```python
from build123d import *

# Parameters (mm, degrees)
BOSS_EXTRUDE3_DEPTH = 4.7625
BOSS_EXTRUDE5_DEPTH = 1.5875
SKETCH12_W          = 6.35
SKETCH12_H          = 35.71875
CUT_EXTRUDE1_DEPTH  = 9.652


with BuildPart() as part:
    # Sketch1 → Boss-Extrude3 (new body)
    with BuildSketch(Plane.XY):
        Polygon((43.795067265, 15.433632287), (5.695067265, 15.433632287), (5.695067265, -60.766367713), (43.795067265, -60.766367713), (43.795067265, -25.047617713), (31.095067265, -25.047617713), (31.095067265, -20.285117713), (43.795067265, -20.285117713), align=None)
    extrude(amount=BOSS_EXTRUDE3_DEPTH)

    # Sketch3 → Boss-Extrude5 (add)
    with BuildSketch(Plane.XY.offset(4.7625)):
        Polygon((18.395067265, -6.791367713), (5.695067265, -6.791367713), (5.695067265, -22.666367713), (5.695067265, -38.541367713), (18.395067265, -38.541367713), align=None)
    extrude(amount=BOSS_EXTRUDE5_DEPTH)

    # Sketch12 → Cut-Extrude1 (cut)
    with BuildSketch(Plane.XY.offset(4.7625)):
        with Locations((40.620067265, -42.906992713)):
            Rectangle(SKETCH12_W, SKETCH12_H)
        with Locations((40.620067265, -2.425742713)):
            Rectangle(SKETCH12_W, SKETCH12_H)
    extrude(amount=-CUT_EXTRUDE1_DEPTH, mode=Mode.SUBTRACT)


solid = part.part
```
CAD build for the part. Positions are in the model's coordinates, mm. A direction names the side the tool comes from. Coordinates: 2 decimals unless noted, no trailing zeros. Loops run counter-clockwise (first coordinate to the right, second up) from the corner with the lowest first, then second, coordinate; pieces in that order, holes last. Notation, with made-up numbers: (48, 56.25) - (97, 56.25) arc R20 cw to (97, 83.25) - close; hole circle Ø1 at (53, 60.25). An arc over 180 degrees is marked (long way). Use CSV: the item, a comma, the result in double quotes. Start each with the question number.
Q1. Cut at A-A, the plane x = 35. List the corners of the cut face in (y, z).
Q2. Cut at C-C, the plane x = 12. List the corners of the cut face in (y, z), then the cut area to 3 significant figures.
Q3. 3-axis set-ups, long thin cutter, end or side, ignore diameter. For faces 5 (the flat face through (12, -38.541, 6)), 6 (the flat face through (12, -6.791, 6)), 7 (the flat face through (18.395, -23, 6)), 8 (the flat face through (31.095, -23, 2)): which of +Z, -Z, +X, -X, +Y, -Y reach the whole face in a straight line?
Q4. Drop flat-ended pins along their axis: P1, Ø0.5, axis at y = -27, z = 5.5, coming from the +X side; P2, Ø0.5, axis at x = 12.5, z = 5.5, coming from the +Y side; P3, Ø0.8, axis at x = 10.5, z = 6, coming from the -Y side. Give the stop position or say it passes through.
Q5. Cut at B-B, the plane y = -22. List the corners of the cut face in (x, z), then the cut area to 3 significant figures.
Q6. Cut at D-D, the plane y = -1. List the corners of the cut face in (x, z).
Q7. Probe probe 1 along Z at (x, y) = (9, -4); probe 2 along Y at (x, z) = (33.5, 3.5); probe 3 along X at (y, z) = (-34.5, 5.5). List the from-to ranges inside material, lowest first. Write a range as from..to.
Q8. Two-plate mould, pull along Y, no slides. Class faces 1 (the flat face through (22, 15.434, 2)), 2 (the flat face through (34, -20.285, 2)), 3 (the flat face through (34, -25.048, 2)), 4 (the flat face through (21, -60.766, 2)): +Y half, -Y half, draft (parallel to the pull), parting line (faces both ways), or undercut.
Here are the results:
1,outline,"(-60.77, 0) - (-25.05, 0) - (-25.05, 4.76) - (-60.77, 4.76) - close; (-20.29, 0) - (15.43, 0) - (15.43, 4.76) - (-20.29, 4.76) - close"
2,outline,"(-60.77, 0) - (15.43, 0) - (15.43, 4.76) - (-6.79, 4.76) - (-6.79, 6.35) - (-38.54, 6.35) - (-38.54, 4.76) - (-60.77, 4.76) - close"
2,area,"413 mm2"
3,face 5,"+Z, +X, -X, -Y"
3,face 6,"+Z, +X, -X, +Y"
3,face 7,"+Z, +X, +Y, -Y"
3,face 8,"+Z, -Z, +X"
4,P1,"x = 18.4"
4,P2,"y = -6.79"
4,P3,"y = -38.54"
5,outline,"(5.7, 0) - (31.1, 0) - (31.1, 4.76) - (18.4, 4.76) - (18.4, 6.35) - (5.7, 6.35) - close"
5,area,"141 mm2"
6,outline,"(5.7, 0) - (37.45, 0) - (37.45, 4.76) - (5.7, 4.76) - close"
7,probe 1,"0..4.76"
7,probe 2,"-60.77..-25.05, -20.29..15.43"
7,probe 3,"5.7..18.4"
8,face 1,"+Y half"
8,face 2,"undercut"
8,face 3,"undercut"
8,face 4,"-Y half"
